```python
from build123d import *

# Parameters (mm, degrees)
BOSS_EXTRUDE1_DEPTH = 6.35
SKETCH2_W           = 18
SKETCH2_H           = 3
CUT_EXTRUDE1_DEPTH  = 148.509567486
CUT_EXTRUDE2_DEPTH  = 3.5
SKETCH8_R           = 1.6
CUT_EXTRUDE3_DEPTH  = 148.509567486


with BuildPart() as part:
    # Sketch1 → Boss-Extrude1 (new body)
    with BuildSketch(Plane(origin=(0, 0, 0), x_dir=(1, 0, 0), z_dir=(0, 1, 0))):
        Polygon((64.951905284, 87.5), (-64.951905284, 87.5), (-108.253175473, 12.5), (-43.301270189, -100), (43.301270189, -100), (108.253175473, 12.5), align=None)
    extrude(amount=BOSS_EXTRUDE1_DEPTH)

    # Sketch2 → Cut-Extrude1 (cut, through all)
    with BuildSketch(Plane(origin=(0, 6.35, 0), x_dir=(1, 0, 0), z_dir=(0, 1, 0))):
        with Locations((-29, -92.2)):
            Rectangle(SKETCH2_W, SKETCH2_H)
        with Locations((29, -92.2)):
            Rectangle(SKETCH2_W, SKETCH2_H)
        Polygon((-62.146580335, 79.758965344), (-59.548504123, 78.258965344), (-68.548504123, 62.670508076), (-71.146580335, 64.170508076), align=None)
        Polygon((-97.548504123, 12.441034656), (-88.548504123, 28.029491924), (-91.146580335, 29.529491924), (-100.146580335, 13.941034656), align=None)
        Polygon((100.146580335, 13.941034656), (91.146580335, 29.529491924), (88.548504123, 28.029491924), (97.548504123, 12.441034656), align=None)
        Polygon((59.548504123, 78.258965344), (62.146580335, 79.758965344), (71.146580335, 64.170508076), (68.548504123, 62.670508076), align=None)
    extrude(amount=-CUT_EXTRUDE1_DEPTH, mode=Mode.SUBTRACT)

    # Sketch4 → Cut-Extrude2 (cut)
    with BuildSketch(Plane(origin=(0, 6.35, 0), x_dir=(1, 0, 0), z_dir=(0, 1, 0))):
        Polygon((-62.631397208, -1.519237886), (32.631397208, 53.480762114), (62.631397208, 1.519237886), (-32.631397208, -53.480762114), align=None)
    extrude(amount=-CUT_EXTRUDE2_DEPTH, mode=Mode.SUBTRACT)

    # Sketch8 → Cut-Extrude3 (cut, through all)
    with BuildSketch(Plane(origin=(0, 6.35, 0), x_dir=(1, 0, 0), z_dir=(0, 1, 0))):
        with Locations(Location((-64.137841404, -37.03, 0), (0, 0, 270))):
            Circle(SKETCH8_R)
        with Locations(Location((64.137841404, -37.03, 0), (0, 0, 270))):
            Circle(SKETCH8_R)
        with Locations(Location((0, 74.06, 0), (0, 0, 270))):
            Circle(SKETCH8_R)
    extrude(amount=-CUT_EXTRUDE3_DEPTH, mode=Mode.SUBTRACT)


solid = part.part
```
Read the model definition and answer for the solid it produces. Units are mm, in the model's axes. A direction names the side the tool comes from. Give positions to 0.01 mm unless a question says otherwise; leave off trailing zeros. Write each loop counter-clockwise with the first axis right and the second up, starting at its lowest first coordinate (ties: lowest second). Pieces come first, ordered by that corner, then holes. Notation, with made-up numbers: M 0,-36 L 32,-36 A14 cw 32,-12 Z; hole C 84,-35 d8. An arc over 180 degrees is marked long. Put each result on its own line as item: value. Start each with the question number.
1. Which of the six approach directions +Z, -Z, +X, -X, +Y, -Y give full straight-line access (tool end or side, diameter ignored) to faces 1 (the flat face through (75.32, 3.13, 44.54)), 2 (the flat face through (-47.4, 4.6, 27.9)), 3 (the flat face through (-63.99, 3.22, -70.57))?
2. Each of these flat-tipped pins is pushed along its axis until it touches: pin 1 Ø2 at (x, y) = (56.5, 2) entering from +Z; pin 2 Ø2.5 at (y, z) = (2, 93) entering from -X; pin 3 Ø3.5 at (y, z) = (1.5, 92.5) entering from +X; pin 4 Ø1.9 at (x, z) = (0, -74.06) entering from +Y. Where does it stop, or does it pass through?
3. The part is cut by section B-B, the plane x = -10. Give the vertices of the cut face in (y, z), and give its area (3 significant figures).
4. The part is cut by section D-D, the plane y = 5. Give the number of separate pieces and of enclosed holes in the cut face, and give its area (3 significant figures).
5. The part is cut by section A-A, the plane x = 29. Give the vertices of the cut face in (y, z).
6. For a pull along X with two mould halves and no side action, classify faces 4 (the flat face through (-86.299, 3.131, -50.525)), 5 (the flat face through (-15.667, 4.624, -25.596)), 6 (the flat face through (-2, 0, 5)) as released by +X, released by -X, zero draft, split by the parting line, or undercut.
7. Consider line 1 along X through (y, z) = (4, -74.06); line 2 along X through (y, z) = (4.5, 37.03); line 3 along Z through (x, y) = (-35, 4.5). Determine where each line is inside the solid, lowest interval first.
8. The part is cut by section C-C, the plane z = 83. Give the vertices of the cut face in (x, y), and give its area (3 significant figures).
Final values:
1. face 1: +Z, +X, +Y, -Y
1. face 2: +Y
1. face 3: +Y, -Y
2. pin 1: stops at z = 78.87
2. pin 2: stops at x = -48.06
2. pin 3: stops at x = 48.64
2. pin 4: passes through
3. outline: M 0,-87.5 L 6.35,-87.5 L 6.35,-28.87 L 2.85,-28.87 L 2.85,40.41 L 6.35,40.41 L 6.35,100 L 0,100 Z
3. area: 948 mm²
4. separate pieces: 1
4. enclosed holes: 10
4. area: 23,100 mm²
5. outline: M 0,-87.5 L 6.35,-87.5 L 6.35,-51.38 L 2.85,-51.38 L 2.85,17.9 L 6.35,17.9 L 6.35,90.7 L 0,90.7 Z; M 0,93.7 L 6.35,93.7 L 6.35,100 L 0,100 Z
6. face 4: released by -X
6. face 5: undercut
6. face 6: zero draft
7. line 1: x = -72.71 to -65.44, -61.97 to -1.6, 1.6 to 61.97, 65.44 to 72.71
7. line 2: x = -79.66 to -65.74, -62.54 to -42.13, -4.14 to 62.54, 65.74 to 79.66
7. line 3: z = -87.5 to -14.43, 49.38 to 90.7, 93.7 to 100
8. outline: M -53.12,0 L 53.12,0 L 53.12,6.35 L -53.12,6.35 Z
8. area: 675 mm²
